from build123d import *

# Parameters (mm, degrees)
SKETCH1_W           = 12.7
SKETCH1_H           = 6.35
BOSS_EXTRUDE1_DEPTH = 6.096
SKETCH2_R           = 3.175
BOSS_EXTRUDE2_DEPTH = 69.85


with BuildPart() as part:
    # Sketch1 → Boss-Extrude1 (new body)
    with BuildSketch(Plane.XY):
        with Locations((6.35, 3.175)):
            Rectangle(SKETCH1_W, SKETCH1_H)
    extrude(amount=BOSS_EXTRUDE1_DEPTH)

    # Sketch2 → Boss-Extrude2 (add)
    with BuildSketch(Plane.XY.offset(6.096)):
        with Locations(Location((6.35, 3.175, 0), (0, 0, 270))):
            Circle(SKETCH2_R)
    extrude(amount=BOSS_EXTRUDE2_DEPTH)

    # Sketch4 → Revolve1 (revolve)
    with BuildSketch(Plane(origin=(6.35, 0, 0), x_dir=(0, 0, -1), z_dir=(1, 0, 0))):
        with BuildLine():
            Line((-75.946, 6.35), (-75.946, 3.175))
            Line((-75.946, 3.175), (-79.121, 3.175))
            ThreePointArc((-79.121, 3.175), (-78.19106403, 5.42006403), (-75.946, 6.35))
        make_face()
    revolve(axis=Axis((6.35, 3.175, -3.95605), (0, 0, 1)))


solid = part.part
CAD build for the part. Positions are in the model's coordinates, mm. A direction names the side the tool comes from. Coordinates: 2 decimals unless noted, no trailing zeros. Write each loop counter-clockwise with the first axis right and the second up, starting at its lowest first coordinate (ties: lowest second). Pieces come first, ordered by that corner, then holes. Notation, with made-up numbers: M 85.25,86 L 108.25,86 A37 cw 108.25,123 Z; hole C 23,32 d5. An arc over 180 degrees is marked long. Return JSON: item names as keys, results as strings.
Item 1: Slice it at A-A, the plane y = 2.25. Write the cut outline in (x, z).
Findings below:
{"outline": "M 0,0 L 12.7,0 L 12.7,6.1 L 9.39,6.1 L 9.39,75.95 A3.04 ccw 3.31,75.95 L 3.31,6.1 L 0,6.1 Z"}
Item 2: Slice it at B-B, the plane x = 4.75. Write the cut outline in (y, z) (3 decimals).
Findings below:
{"outline": "M 0,0 L 6.35,0 L 6.35,6.096 L 5.917,6.096 L 5.917,75.946 A2.742 ccw 0.433,75.946 L 0.433,6.096 L 0,6.096 Z"}
Item 3: Drop flat-ended pins along their axis: pin 1 Ø1.9 at (x, y) = (10.5, 2) entering from +Z; pin 2 Ø3 at (x, y) = (5.5, 2) entering from -Z; pin 3 Ø3 at (x, y) = (9, 1.5) entering from +Z; pin 4 Ø1 at (y, z) = (4, 29.5) entering from +X. Give the stop position or say it passes through.
Findings below:
{"pin 1": "stops at z = 6.1", "pin 2": "stops at z = 0", "pin 3": "stops at z = 78.67", "pin 4": "stops at x = 9.51"}
Item 4: Slice it at C-C, the plane z = 29. Write the cut outline in (x, y) (3 decimals), and give its area (3 significant figures).
Findings below:
{"outline": "C 6.35,3.175 d6.35", "area": "31.7 mm2"}
Item 5: Probe line 1 (Z direction, x = 3.25, y = 5.75); line 2 (X direction, y = 3.5, z = 70); line 3 (Z direction, x = 4.25, y = 4.25). List the from-to ranges inside material, lowest first. Write a range as from..to.
Findings below:
{"line 1": "z = 0..6.1", "line 2": "x = 3.19..9.51", "line 3": "z = 0..78.07"}
Item 6: Which spindle directions (+Z, -Z, +X, -X, +Y, -Y) get a long thin tool onto all of the face, cutting with end or side? Do faces 1 (the cylindrical face through (9.03, 1.47, 40.53)), 2 (the flat face through (0, 3, 3)), 3 (the flat face through (11, 3, 6.096)). Say none if no direction does.
Findings below:
{"face 1": "+Z", "face 2": "+Z, -Z, -X, +Y, -Y", "face 3": "+Z, +X"}
